The model under review builds one solid part; all positions refer to its coordinate system, in mm. Face numbers are marked on the shaded views. A direction names the side the tool comes from. Coordinates: 2 decimals unless noted, no trailing zeros. Loops run counter-clockwise (first coordinate to the right, second up) from the corner with the lowest first, then second, coordinate; pieces in that order, holes last. Notation, with made-up numbers: M 71,60.5 L 96,60.5 A25 cw 96,79.5 Z; hole C 5.25,23.5 d2. An arc over 180 degrees is marked long. Return JSON: item names as keys, results as strings.
Autodesk Inventor part; units mm, degrees
ref_plane "YZ Plane" through (0, 0, 0) normal (1, 0, 0) x (0, 1, 0)
ref_plane "XZ Plane" through (0, 0, 0) normal (0, 1, 0) x (-1, 0, 0)
ref_plane "XY Plane" through (0, 0, 0) normal (0, 0, 1) x (1, 0, 0)
sketch "Sketch1" plane through (0, 0, 0) normal (0, 0, 1) x (1, 0, 0)
  line L0 (-4, 16) -> (4, 16)
  line L1 (4, 16) -> (4, -16)
  line L2 (4, -16) -> (-4, -16)
  line L3 (-4, -16) -> (-4, 16)
  point P0 (0, 0)
  dimension "d0" = 8
  dimension "d1" = 32
  dimension "d2" = 4
  dimension "d3" = 16
extrude "Extrusion1" add sketch "Sketch1" along normal blind 3.2
shell "Shell1" thickness 1.5 removed faces 1 at (-1.3333, 5.3333, 0)
sketch "Sketch2" plane through (0, 0, 3.2) normal (0, 0, 1) x (1, 0, 0)
  circle A0 centre (0, -12) radius 2.5
  line L0 (4, 16) -> (4, -16)
  line L1 (4, -16) -> (-4, -16)
  dimension "d7" = 5
  dimension "d10" = 4
  dimension "d11" = 4
extrude "Extrusion2" add sketch "Sketch2" along normal blind 1.6
sketch "Sketch3" plane through (2.5, -14.5, 1.7) normal (0, 0, -1) x (-1, 0, 0)
  circle A0 centre (2.5, 2.5) radius 2.5
  circle A1 centre (2.5, 2.5) radius 1.2
  point P0 (2.5, 14.5)
  dimension "d18" = 2.4
extrude "Extrusion3" cut sketch "Sketch3" against normal blind 1.6 contours A1
pattern_linear "Rectangular Pattern1" count 4 spacing 8 along (0, 1, 0) of "Extrusion2", "Extrusion3"
sketch "Sketch4" plane through (2.5, -14.5, 1.7) normal (0, 0, -1) x (-1, 0, 0)
  circle A0 centre (2.5, 10.5) radius 1.2
  circle A1 centre (2.5, 2.5) radius 1.2
  line L0 (0, 29) -> (0, 0)
  line L1 (0, 0) -> (5, 0)
  circle A2 centre (6.5, 6.5) radius 3.15
  circle A3 centre (6.5, 6.5) radius 2.5
  point P0 (2.5, 14.5)
  dimension "d21" = 6.5
  dimension "d22" = 6.5
  dimension "d23" = 10.5
  dimension "d24" = 2.5
  dimension "d25" = 5
  dimension "d26" = 6.3
extrude "Extrusion4" [suppressed]
pattern_linear "Rectangular Pattern2" [suppressed]
equation "\"d0\" = 0.8 * WIDTH"
equation "\"d1\" = 0.8 * LENGTH"
equation "\"d4\" = HEIGHT"
equation "\"d21\" = 0.5 * d23 + 0.5 * d24"
equation "\"d22\" = d21"
equation "\"WIDTH\" = 1"
equation "\"HEIGHT\" = 3.2"
properties part number "3710" material "Steel"
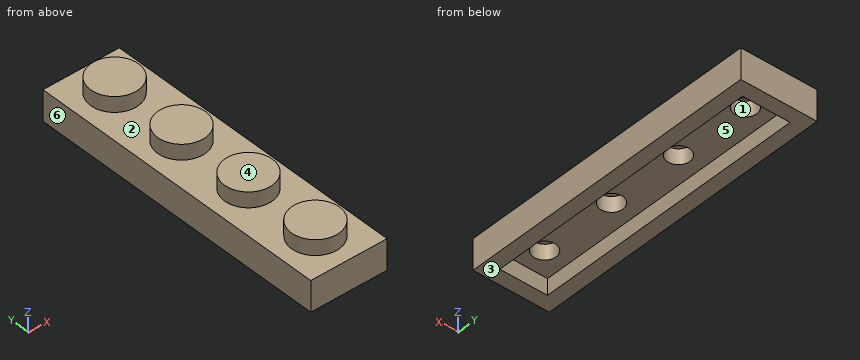
1. Add section B-B on y = 2. Give the boundary of the cut face in (x, z), plus the area to 3 significant figures.
Check values:
{"outline": "M -4,0 L -2.5,0 L -2.5,1.7 L 2.5,1.7 L 2.5,0 L 4,0 L 4,3.2 L 1.5,3.2 L 1.5,4.8 L -1.5,4.8 L -1.5,3.2 L -4,3.2 Z", "area": "21.9 mm²"}
2. Add section C-C on z = 2.65. Give the boundary of the cut face in (x, y).
Check values:
{"outline": "M -4,-16 L 4,-16 L 4,16 L -4,16 Z; hole C 0,-12 d2.4; hole C 0,-4 d2.4; hole C 0,4 d2.4; hole C 0,12 d2.4"}
3. Add section A-A on z = 1.3. Give the boundary of the cut face in (x, y).
Check values:
{"outline": "M -4,-16 L 4,-16 L 4,16 L -4,16 Z; hole M -2.5,-14.5 L 2.5,-14.5 L 2.5,14.5 L -2.5,14.5 Z"}
4. To check wall thickness, follow line 1 (Y direction, x = 0, z = 2.85); line 2 (X direction, y = -13, z = 0.4); line 3 (Y direction, x = 0, z = 4.05). State the ranges of each line that lie inside material, in increasing order.
Check values:
{"line 1": "-16 to -13.2, -10.8 to -5.2, -2.8 to 2.8, 5.2 to 10.8, 13.2 to 16", "line 2": "-4 to -2.5, 2.5 to 4", "line 3": "-14.5 to -9.5, -6.5 to -1.5, 1.5 to 6.5, 9.5 to 14.5"}
5. Add section D-D on y = -4. Give the boundary of the cut face in (x, z).
Check values:
{"outline": "M -4,0 L -2.5,0 L -2.5,1.7 L -1.2,1.7 L -1.2,3.3 L 1.2,3.3 L 1.2,1.7 L 2.5,1.7 L 2.5,0 L 4,0 L 4,3.2 L 2.5,3.2 L 2.5,4.8 L -2.5,4.8 L -2.5,3.2 L -4,3.2 Z"}
6. Insertion check: pin 1 Ø2.5 at (x, y) = (0.5, 4.5) entering from -Z; pin 2 Ø1.9 at (x, y) = (0, -12) entering from -Z; pin 3 Ø3 at (x, y) = (2, -7.5) entering from +Z. Each pin has a flat end and moves straight along its axis. Give the tip position at first contact, or say it passes through.
Check values:
{"pin 1": "z = 1.7", "pin 2": "z = 3.3", "pin 3": "z = 3.2"}
7. Machinability: for the marked faces 1, 2 and 3, which of the approach directions +Z, -Z, +X, -X, +Y, -Y give a long, thin tool a straight path to every point of the face, cutting with its end or side? Answer none if there is none.
Check values:
{"face 1": "-Z", "face 2": "+Z", "face 3": "-Z, +X, -X, +Y, -Y"}
8. The part is to be moulded in two halves that separate along X. For the marked faces 4, 5 and 6, say which applies: released by +X, released by -X, zero draft, split by the parting line, or undercut.
Check values:
{"face 4": "zero draft", "face 5": "undercut", "face 6": "released by -X"}
